from build123d import *

# Parameters (mm, degrees)
EXTRUDE_1_DEPTH     = 4
SKETCH_2_R          = 2.025
CUT_EXTRUDE_1_DEPTH = 5
SKETCH_3_W          = 18
SKETCH_3_H          = 18
CUT_EXTRUDE_2_DEPTH = 5
FILLET_1_R          = 2
FILLET_2_R          = 3


with BuildPart() as part:
    # 草图1 → 凸台-拉伸1 (new body)
    with BuildSketch(Plane.XY):
        Polygon((0, 0), (0, -90), (-30, -90), (-50, -30), (-50, 0), align=None)
    extrude(amount=EXTRUDE_1_DEPTH)

    # 草图2 → 切除-拉伸1 (cut, through all)
    with BuildSketch(Plane.XY.offset(4)):
        with Locations((-15, -75)):
            Circle(SKETCH_2_R)
        with Locations((-15, -45)):
            Circle(SKETCH_2_R)
        with Locations((-15, -15)):
            Circle(SKETCH_2_R)
        with Locations((-40, -15)):
            Circle(SKETCH_2_R)
    extrude(amount=-CUT_EXTRUDE_1_DEPTH, mode=Mode.SUBTRACT)

    # 草图3 → 切除-拉伸2 (cut, through all)
    with BuildSketch(Plane.XY.offset(4)):
        Polygon((-44.729537233, -30), (-30, -30), (-30, -74.188611699), align=None)
        with Locations((-15, -30)):
            Rectangle(SKETCH_3_W, SKETCH_3_H)
        with Locations((-15, -60)):
            Rectangle(SKETCH_3_W, SKETCH_3_H)
    extrude(amount=-CUT_EXTRUDE_2_DEPTH, mode=Mode.SUBTRACT)

    # 圆角1
    fillet_1_edges = [part.edges().sort_by_distance(p)[0] for p in [
        (-30, -74.188611699, 2),
        (-44.729537233, -30, 2),
        (-30, -30, 2),
        (-6, -51, 2),
        (-6, -69, 2),
        (-24, -69, 2),
        (-24, -51, 2),
        (-6, -21, 2),
        (-6, -39, 2),
        (-24, -39, 2),
        (-24, -21, 2),
    ]]
    fillet(fillet_1_edges, radius=FILLET_1_R)

    # 圆角2
    fillet_2_edges = [part.edges().sort_by_distance(p)[0] for p in [
        (0, 0, 2),
        (0, -90, 2),
        (-30, -90, 2),
        (-50, -30, 2),
        (-50, 0, 2),
    ]]
    fillet(fillet_2_edges, radius=FILLET_2_R)


solid = part.part
The model under review builds one solid part; all positions refer to its coordinate system, in mm. A direction names the side the tool comes from. Give positions to 0.01 mm unless a question says otherwise; leave off trailing zeros. Order: outer loops, then holes, each group sorted by start corner. A loop starts at its lowest first (then second) coordinate and runs counter-clockwise, first axis right, second up. Notation, with made-up numbers: M 5,18.5 L 62,18.5 A27 ccw 62,54.5 Z; hole C 7,19 d9. An arc over 180 degrees is marked long. Answer in a Markdown table with one row per item. Add a question column.
1. To check wall thickness, follow line 1 along Y through (x, z) = (-17.5, 3.3); line 2 along Y through (x, z) = (-15, 1.75) (3 decimals); line 3 along X through (y, z) = (-24.5, 1.3). State the ranges of each line that lie inside material, in increasing order.
2. Mouldability with a two-part tool opening along X and no side actions: class faces 3 (the cylindrical face through (-0.86, -0.9, 2.03)), 4 (the cylindrical face through (-29.57, -89.45, 2.03)), 5 (the flat face through (-38.805, -47.774, 2.028)) as released by +X, released by -X, zero draft, split by the parting line, or undercut.
3. Add section D-D on y = -75. State the section outline as (x, z) points (3 decimals).
4. Add section B-B on x = -10. State the section outline as (y, z) points, plus the area to 3 significant figures.
5. Machinability: for faces 1 (the flat face through (-25, -44, 0)), 2 (the cylindrical face through (-23.4, -21.57, 1.97)), which of the approach directions +Z, -Z, +X, -X, +Y, -Y give a long, thin tool a straight path to every point of the face, cutting with its end or side? Answer none if there is none.
6. Add section C-C on y = -15. State the section outline as (x, z) points (3 decimals).
7. Add section A-A on y = -24.5. State the section outline as (x, z) points, plus the area to 3 significant figures.
8. For pin 1 Ø2.5 at (x, y) = (-15, -45) entering from -Z; pin 2 Ø2 at (y, z) = (-60.5, 2.5) entering from -X; pin 3 Ø1.2 at (y, z) = (-48.5, 1.5) entering from -X, all flat-tipped, find the tip position at first contact; note any pin that passes through.
The answers:
| question | item | result |
|---|---|---|
| 1 | line 1 | -90 to -69, -51 to -39, -21 to 0 |
| 1 | line 2 | -90 to -77.025, -72.975 to -69, -51 to -47.025, -42.975 to -39, -21 to -17.025, -12.975 to 0 |
| 1 | line 3 | -50 to -24, -6 to 0 |
| 2 | face 3 | released by +X |
| 2 | face 4 | released by -X |
| 2 | face 5 | undercut |
| 3 | outline | M -35,0 L -17.025,0 L -17.025,4 L -35,4 Z; M -12.975,0 L 0,0 L 0,4 L -12.975,4 Z |
| 4 | outline | M -90,0 L -69,0 L -69,4 L -90,4 Z; M -51,0 L -39,0 L -39,4 L -51,4 Z; M -21,0 L 0,0 L 0,4 L -21,4 Z |
| 4 | area | 216 mm2 |
| 5 | face 1 | -Z, +X, -X, +Y, -Y |
| 5 | face 2 | +Z, -Z |
| 6 | outline | M -50,0 L -42.025,0 L -42.025,4 L -50,4 Z; M -37.975,0 L -17.025,0 L -17.025,4 L -37.975,4 Z; M -12.975,0 L 0,0 L 0,4 L -12.975,4 Z |
| 7 | outline | M -50,0 L -24,0 L -24,4 L -50,4 Z; M -6,0 L 0,0 L 0,4 L -6,4 Z |
| 7 | area | 128 mm2 |
| 8 | pin 1 | through |
| 8 | pin 2 | x = -40.17 |
| 8 | pin 3 | x = -44.03 |
